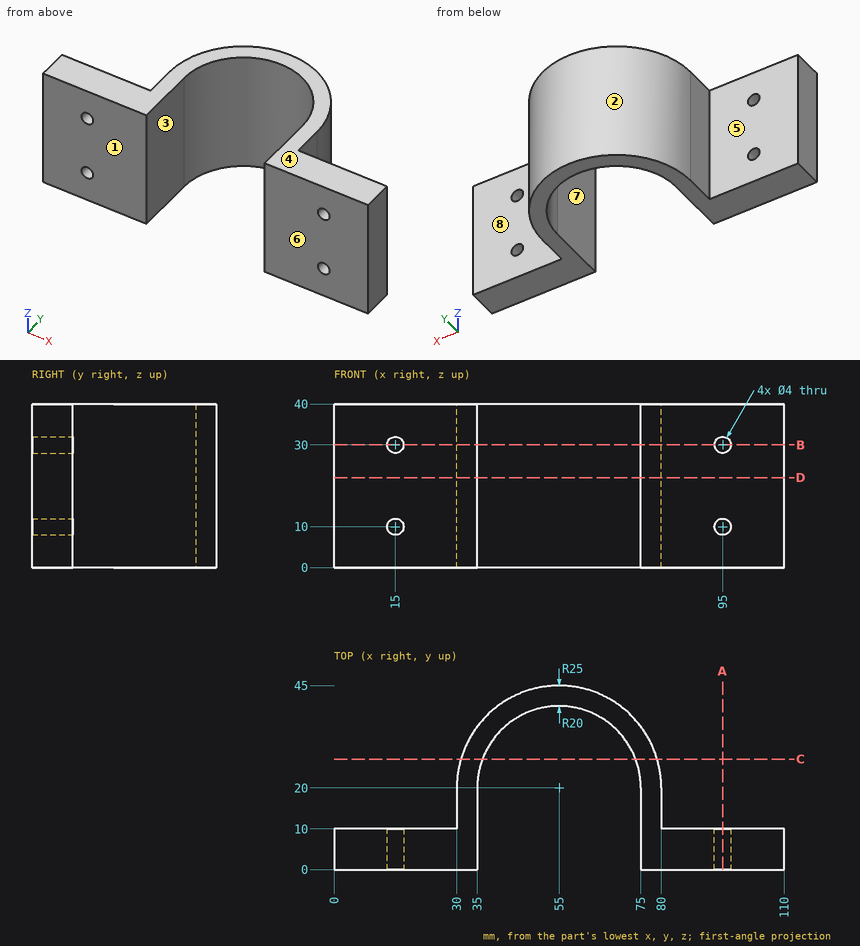
Part print with two shaded views. Sizes in mm from the minimum x, y, z corner. A direction names the side the tool comes from. Coordinates: 2 decimals unless noted, no trailing zeros. Loops run counter-clockwise (first coordinate to the right, second up) from the corner with the lowest first, then second, coordinate; pieces in that order, holes last. Notation, with made-up numbers: M 29.25,46 L 83.25,46 A18 ccw 83.25,76 Z; hole C 29,-25 d9. An arc over 180 degrees is marked long. Use CSV: the item, a comma, the result in double quotes. Start each with the question number.
1. Tool access for the marked faces 4, 5, 6, 7 and 8: list every direction of +Z, -Z, +X, -X, +Y, -Y with a clear straight run to the whole face (end or side of a thin tool).
2. Band-saw the part on C-C, the plane y = 27. List the corners of the cut face in (x, z) (3 decimals).
3. Two-plate mould, pull along X, no slides. Class the marked faces 1, 2 and 3: pulls with the +X half, pulls with the -X half, needs draft (parallel to the pull), parting line crosses it, or undercut.
4. Flat gauge pins, fed straight in: pin 1 (2.5 mm diameter, centred on x = 15, z = 10, fed in from +Y); pin 2 (12 mm diameter, centred on x = 34.5, y = 5, fed in from -Z); pin 3 (6.5 mm diameter, centred on x = 95, z = 30, fed in from +Y); pin 4 (6 mm diameter, centred on y = 21, z = 16.5, fed in from -X). Where does each tip first touch, or does it go through?
5. Band-saw the part on B-B, the plane z = 30. List the corners of the cut face in (x, y).
6. Band-saw the part on A-A, the plane x = 95. List the corners of the cut face in (y, z), then the cut area to 3 significant figures.
7. Probe probe 1 along Z at (x, y) = (15, 4); probe 2 along X at (y, z) = (4.5, 10); probe 3 along X at (y, z) = (17, 19). List the from-to ranges inside material, lowest first. Write a range as [from, to].
8. Band-saw the part on D-D, the plane z = 22. List the corners of the cut face in (x, y), then the cut area to 3 significant figures.
Entries:
1,face 4,"+Z, +X, -X, +Y, -Y"
1,face 5,"+Z, -Z, -X, +Y"
1,face 6,"+Z, -Z, +X, -X, -Y"
1,face 7,"+Z, -Z, -Y"
1,face 8,"+Z, -Z, +X, +Y"
2,outline,"M 31,0 L 36.265,0 L 36.265,40 L 31,40 Z; M 73.735,0 L 79,0 L 79,40 L 73.735,40 Z"
3,face 1,"needs draft"
3,face 2,"parting line crosses it"
3,face 3,"undercut"
4,pin 1,"passes through"
4,pin 2,"stops at z = 0"
4,pin 3,"stops at y = 10"
4,pin 4,"stops at x = 30"
5,outline,"M 0,0 L 13,0 L 13,10 L 0,10 Z; M 17,0 L 35,0 L 35,20 A20 cw 75,20 L 75,0 L 93,0 L 93,10 L 80,10 L 80,20 A25 ccw 30,20 L 30,10 L 17,10 Z; M 97,0 L 110,0 L 110,10 L 97,10 Z"
6,outline,"M 0,0 L 10,0 L 10,8 L 0,8 Z; M 0,12 L 10,12 L 10,28 L 0,28 Z; M 0,32 L 10,32 L 10,40 L 0,40 Z"
6,area,"320 mm2"
7,probe 1,"z = [0, 8], [12, 28], [32, 40]"
7,probe 2,"x = [0, 13], [17, 35], [75, 93], [97, 110]"
7,probe 3,"x = [30, 35], [75, 80]"
8,outline,"M 0,0 L 35,0 L 35,20 A20 cw 75,20 L 75,0 L 110,0 L 110,10 L 80,10 L 80,20 A25 ccw 30,20 L 30,10 L 0,10 Z"
8,area,"1,150 mm2"
